Input: part model. Units: mm. Frame: model coordinates. A direction names the side the tool comes from. Give positions to 0.01 mm unless a question says otherwise; leave off trailing zeros. Loops run counter-clockwise (first coordinate to the right, second up) from the corner with the lowest first, then second, coordinate; pieces in that order, holes last. Notation, with made-up numbers: M -22.5,21.5 L 25.5,21.5 A18 ccw 25.5,53.5 Z; hole C 60.5,84 d10. An arc over 180 degrees is marked long. Use a Markdown table: item, result. Add a question column.
from build123d import *

# Parameters (mm, degrees)
SKETCH1_R           = 22.75
SKETCH1_R_2         = 3
BOSS_EXTRUDE1_DEPTH = 25.5
CUT_EXTRUDE1_DEPTH  = 6


with BuildPart() as part:
    # Sketch1 → Boss-Extrude1 (new body)
    with BuildSketch(Plane(origin=(0, 0, 0), x_dir=(1, 0, 0), z_dir=(0, 1, 0))):
        with Locations(Location((0, 0, 0), (0, 0, 270))):
            Circle(SKETCH1_R)
        with Locations(Location((0, 0, 0), (0, 0, 270))):
            Circle(SKETCH1_R_2, mode=Mode.SUBTRACT)
    extrude(amount=BOSS_EXTRUDE1_DEPTH)

    # Sketch2 → Cut-Extrude1 (cut)
    with BuildSketch(Plane(origin=(0, 25.5, 0), x_dir=(1, 0, 0), z_dir=(0, 1, 0))):
        Polygon((5.1, 0), (2.55, 4.416729559), (-2.55, 4.416729559), (-5.1, 0), (-2.55, -4.416729559), (2.55, -4.416729559), align=None)
    extrude(amount=-CUT_EXTRUDE1_DEPTH, mode=Mode.SUBTRACT)


solid = part.part
1) Contact query for flat-ended pins moving along their axis: P1, Ø4, axis at x = -1, y = 21.5, coming from the -Z side; P2, Ø1, axis at x = -10, y = 19, coming from the -Z side; P3, Ø5, axis at x = 17.5, y = 18.5, coming from the +Z side; P4, Ø5.5, axis at x = 0, z = 0, coming from the -Y side. Output: stop coordinate, or through.
2) Section query A-A, the plane y = 12.75. Return the cut outline in (x, z).
3) Reachability of faces 4 (the flat face through (0, 0, 5)), 5 (the flat face through (-3.84, 22.54, 2.18)) from +Z, -Z, +X, -X, +Y, -Y: full face, straight path, thin tool, end or side. Return the list, or none.
4) Section query B-B, the plane x = -17.5. Return the cut outline in (y, z).
5) Section query C-C, the plane z = 10.5. Return the cut outline in (x, y), and give its area (3 significant figures).
6) Pull-direction query (Z, two-part tool) for faces 1 (the flat face through (0, 25.5, 5)), 2 (the cylindrical face through (-13.843, 12.572, -18.054)), 3 (the flat face through (0, 23, -4.417)); classes: pulls with the +Z half, pulls with the -Z half, needs draft (parallel to the pull), parting line crosses it, or undercut.
7) Ray query, line 1 (X direction, y = 9, z = 0); line 2 (Z direction, x = -2, y = 4); line 3 (X direction, y = 10.25, z = 1). Return the intervals inside material, ascending. Write a range as [from, to].
Entries:
| question | item | result |
|---|---|---|
| 1 | P1 | stops at z = -22.75 |
| 1 | P2 | stops at z = -20.67 |
| 1 | P3 | stops at z = 17.1 |
| 1 | P4 | passes through |
| 2 | outline | C 0,0 d45.5; hole C 0,0 d6 |
| 3 | face 4 | +Z, -Z, +X, -X, -Y |
| 3 | face 5 | +Y |
| 4 | outline | M 0,-14.54 L 25.5,-14.54 L 25.5,14.54 L 0,14.54 Z |
| 5 | outline | M -20.18,0 L 20.18,0 L 20.18,25.5 L -20.18,25.5 Z |
| 5 | area | 1,030 mm² |
| 6 | face 1 | needs draft |
| 6 | face 2 | parting line crosses it |
| 6 | face 3 | undercut |
| 7 | line 1 | x = [-22.75, -3], [3, 22.75] |
| 7 | line 2 | z = [-22.66, -2.24], [2.24, 22.66] |
| 7 | line 3 | x = [-22.73, -2.83], [2.83, 22.73] |
